Job drawing, mm, ordinate dimensions from the low corner. One solid piece. A direction names the side the tool comes from. Round coordinates to 2 decimals unless told otherwise and drop trailing zeros. Loops run counter-clockwise (first coordinate to the right, second up) from the corner with the lowest first, then second, coordinate; pieces in that order, holes last. Notation, with made-up numbers: M 6.25,59.25 L 65.25,59.25 A23 cw 65.25,76.25 Z; hole C 56,0.5 d11. An arc over 180 degrees is marked long. Use one line per item in the form item = value. Start each with the question number.
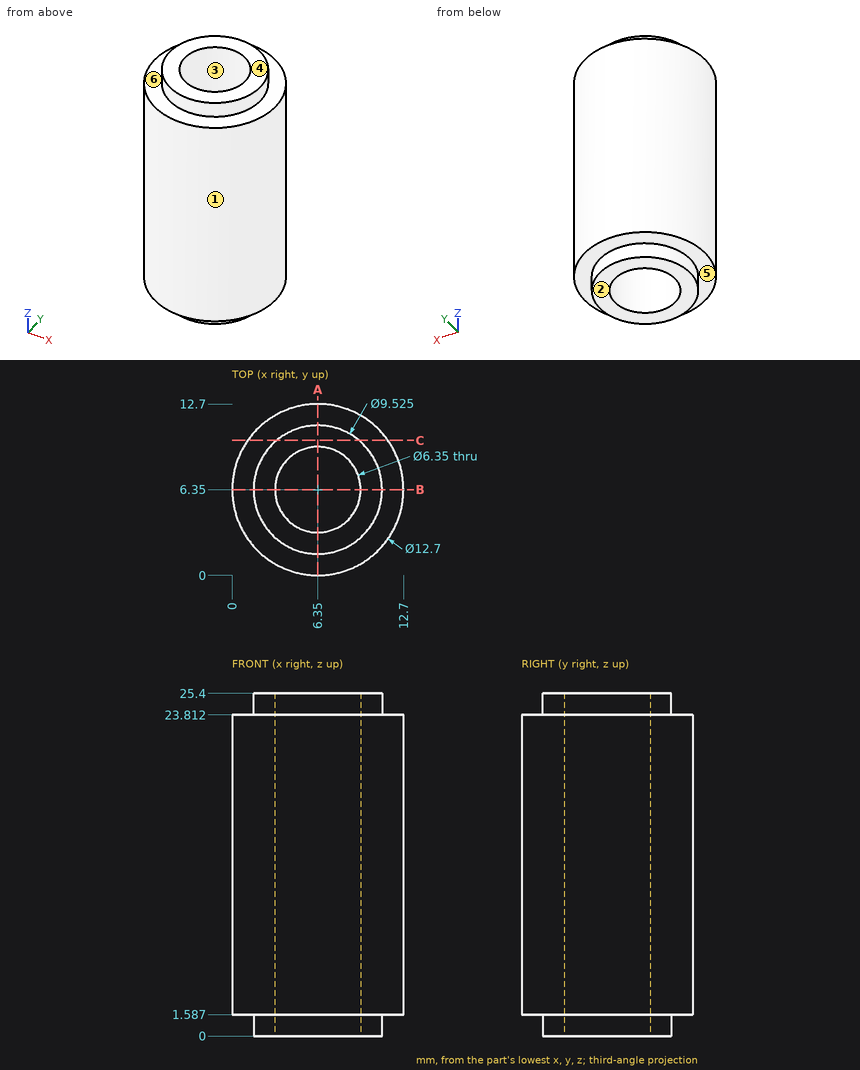
Q1. Pull direction X, two halves, no side cores. Call the marked faces 1, 2 and 3: pulls with the +X half, pulls with the -X half, needs draft (parallel to the pull), parting line crosses it, or undercut.
Q2. Saw through at A-A (x = 6.35). Give the cut face in (y, z) (1 decimal), and give its area (3 significant figures).
Q3. Wall check: probe 1 along Y at (x, z) = (6.35, 14.5) (1 decimal); probe 2 along Z at (x, y) = (11, 7.75); probe 3 along Y at (x, z) = (8.25, 6.25) (1 decimal). Give the ranges that are in metal, low to high.
Q4. Saw through at C-C (y = 10). Give the cut face in (x, z).
Q5. Tool access for the marked faces 4, 5 and 6: list every direction of +Z, -Z, +X, -X, +Y, -Y with a clear straight run to the whole face (end or side of a thin tool).
Q6. Drop flat-ended pins along their axis: P1, Ø1.5, axis at x = 6, y = 3, coming from the -Z side; P2, Ø6, axis at y = 1.5, z = 12.5, coming from the +X side (1 decimal); P3, Ø4, axis at x = 3, z = 14, coming from the -Y side (1 decimal); P4, Ø3, axis at x = 8, z = 8.5, coming from the +Y side. Give the stop position or say it passes through.
Filled in:
q1.face_1 = parting line crosses it
q1.face_2 = needs draft
q1.face_3 = undercut
q2.outline = M 0,1.6 L 1.6,1.6 L 1.6,0 L 3.2,0 L 3.2,25.4 L 1.6,25.4 L 1.6,23.8 L 0,23.8 Z; M 9.5,0 L 11.1,0 L 11.1,1.6 L 12.7,1.6 L 12.7,23.8 L 11.1,23.8 L 11.1,25.4 L 9.5,25.4 Z
q2.area = 151 mm²
q3.probe_1 = 0 to 3.2, 9.5 to 12.7
q3.probe_2 = 1.59 to 23.81
q3.probe_3 = 0.3 to 3.8, 8.9 to 12.4
q4.outline = M 1.15,1.59 L 3.29,1.59 L 3.29,0 L 9.41,0 L 9.41,1.59 L 11.55,1.59 L 11.55,23.81 L 9.41,23.81 L 9.41,25.4 L 3.29,25.4 L 3.29,23.81 L 1.15,23.81 Z
q5.face_4 = +Z, +X, -X, +Y, -Y
q5.face_5 = -Z
q5.face_6 = +Z
q6.P1 = 0
q6.P2 = 12.4
q6.P3 = 0.1
q6.P4 = 12.7
